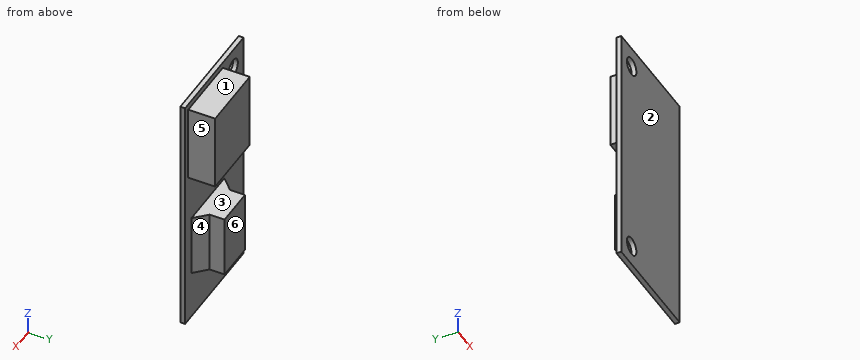
Autodesk Inventor part; units mm, degrees
ref_plane "YZ Plane" through (0, 0, 0) normal (1, 0, 0) x (0, 1, 0)
ref_plane "XZ Plane" through (0, 0, 0) normal (0, 1, 0) x (-1, 0, 0)
ref_plane "XY Plane" through (0, 0, 0) normal (0, 0, 1) x (1, 0, 0)
sketch "Sketch1" plane through (0, 0, 0) normal (0, 1, 0) x (-1, 0, 0)
  line L0 (0, 0) -> (-18.6, 0)
  line L1 (-18.6, 0) -> (-18.6, -41.3)
  line L2 (-18.6, -41.3) -> (0, -41.3)
  line L3 (0, -41.3) -> (0, 0)
  line L4 (-1.8, 0) -> (-1.8, -41.3)
  line L5 (0, -39.35) -> (-18.6, -39.35)
  circle A0 centre (-3.3, -3.45) radius 1.5
  circle A1 centre (-3.3, -37.85) radius 1.5
  line L6 (-8.1, -22.5) -> (-14.6, -22.5)
  line L7 (-14.6, -22.5) -> (-14.6, -33)
  line L8 (-14.6, -33) -> (-8.1, -33)
  line L9 (-8.1, -33) -> (-8.1, -22.5)
  line L10 (-6.6, -1) -> (-17.6, -1)
  line L11 (-17.6, -1) -> (-17.6, -14)
  line L12 (-17.6, -14) -> (-6.6, -14)
  line L13 (-6.6, -14) -> (-6.6, -1)
  line L14 (0, -1.95) -> (-18.6, -1.95)
  dimension "d0" = 18.6
  dimension "d1" = 41.3
  dimension "d2" = 1.8
  dimension "d4" = 1.95
  dimension "d5" = 3
  dimension "d6" = 3
  dimension "d7" = 6.5
  dimension "d8" = 10.5
  dimension "d11" = 8.1
  dimension "d12" = 8.3
  dimension "d13" = 11
  dimension "d14" = 13
  dimension "d16" = 1
  dimension "d17" = 1
  dimension "d27" = 1.95
extrude "Extrusion1" add sketch "Sketch1" against normal blind 0.8 contours L3 L14 L4 L0 | L4 L14 L13 L10 L11 L1 L0 | L3 L5 L4 L14 | L4 A0 L14 | L3 L2 L4 L5 | L14 L11 L12 L13 A0 L4 A1 L5 L1 | L5 A1 L4 | L4 L2 L1 L5 | L14 L13 L12 L11 | L11 L10 L13 L14 | L9 L8 L7 L6
extrude "Extrusion2" add sketch "Sketch1" along normal blind 4.5 contours L14 L13 L12 L11 | L11 L10 L13 L14
extrude "Extrusion3" add sketch "Sketch1" along normal blind 4.5 contours L9 L8 L7 L6
chamfer "Chamfer1" distance 2 angle 45 2 edges at (8.1, 0, -27.75) (14.6, 0, -27.75)
properties part number "interface_board"
Here's how the part is built. I have some questions about the finished solid (model axes, mm). Face numbers are marked on the shaded views. A direction names the side the tool comes from. Give positions to 0.01 mm unless a question says otherwise; leave off trailing zeros. Write each loop counter-clockwise with the first axis right and the second up, starting at its lowest first coordinate (ties: lowest second). Pieces come first, ordered by that corner, then holes. Notation, with made-up numbers: (-33.5, 52.25) -> (-18.5, 52.25) arc R36 ccw to (-18.5, 91.25) -> close; hole circle Ø10 at (-17.5, -27). An arc over 180 degrees is marked (long way). Write each question's results on one line, items separated by ' | '.
Item 1: Suppose I cut it at B-B on x = 9.75. Write out the boundary of the cut face in (y, z), plus the area to 3 significant figures.
Output:
outline: (-0.8, -41.3) -> (0, -41.3) -> (0, -33) -> (4.5, -33) -> (4.5, -22.5) -> (0, -22.5) -> (0, -14) -> (4.5, -14) -> (4.5, -1) -> (0, -1) -> (0, 0) -> (-0.8, 0) -> close | area: 139 mm^2
Item 2: We'd pull the mould along Z, two halves only. Please class the marked faces 1, 2 and 3: pulls with the +Z half, pulls with the -Z half, needs draft (parallel to the pull), parting line crosses it, or undercut.
Output:
face 1: pulls with the +Z half | face 2: needs draft | face 3: undercut
Item 3: For pin 1 Ø1.4 at (x, y) = (10, 2) entering from -Z; pin 2 Ø1.5 at (x, y) = (12.5, 2) entering from +Z; pin 3 Ø1.8 at (x, z) = (3.3, -37.85) entering from -Y; pin 4 Ø2 at (y, z) = (1.5, -8) entering from -X, each with a flat end and sliding along its axis, tell me the tip position at first contact or that it passes through.
Output:
pin 1: stops at z = -33 | pin 2: stops at z = -1 | pin 3: passes through | pin 4: stops at x = 6.6
Item 4: Suppose I cut it at D-D on x = 3.3. Write out the boundary of the cut face in (y, z).
Output:
outline: (-0.8, -41.3) -> (0, -41.3) -> (0, -39.35) -> (-0.8, -39.35) -> close; (-0.8, -36.35) -> (0, -36.35) -> (0, -4.95) -> (-0.8, -4.95) -> close; (-0.8, -1.95) -> (0, -1.95) -> (0, 0) -> (-0.8, 0) -> close
Item 5: If I drill on L1, parallel to Z at x = 3.3, y = -0.15; L2, parallel to X at y = -0.55, z = -3.45; L3, parallel to Z at x = 10, y = 2.1, over which ranges is the centre line in solid material (lowest first)?
Output:
L1: z = -41.3 to -39.35, -36.35 to -4.95, -1.95 to 0 | L2: x = 0 to 1.8, 4.8 to 18.6 | L3: z = -33 to -22.5, -14 to -1
Item 6: Suppose I cut it at A-A on y = 3.5. Write out the boundary of the cut face in (x, z), plus the area to 3 significant figures.
Output:
outline: (6.6, -14) -> (17.6, -14) -> (17.6, -1) -> (6.6, -1) -> close; (8.1, -33) -> (14.6, -33) -> (14.6, -22.5) -> (8.1, -22.5) -> close | area: 211 mm^2
Item 7: On a 3-axis mill with a long thin cutter (end or side, diameter ignored), from which of +Z, -Z, +X, -X, +Y, -Y can I reach the whole of each face in a straight line? I mean the marked faces 4, 5 and 6. Say none if no direction works.
Output:
face 4: -Z, +X, +Y | face 5: +Z, -Z, +X, +Y | face 6: +Z, -Z, +X, -X, +Y
Item 8: Suppose I cut it at C-C on z = -37.85. Write out the boundary of the cut face in (x, y).
Output:
outline: (0, -0.8) -> (1.8, -0.8) -> (1.8, 0) -> (0, 0) -> close; (4.8, -0.8) -> (18.6, -0.8) -> (18.6, 0) -> (4.8, 0) -> close
